```python
from build123d import *

# Parameters (mm, degrees)
BOSS_EXTRUDE1_DEPTH = 107.00004
SKETCH2_R           = 2
CUT_EXTRUDE1_DEPTH  = 16


with BuildPart() as part:
    # Sketch1 → Boss-Extrude1 (new body)
    with BuildSketch(Plane.XY):
        with BuildLine():
            Line((-6.5, 0), (6.5, 0))
            Line((6.5, 0), (6.5, 5.2))
            Line((6.5, 5.2), (4.8, 6.9))
            Line((4.8, 6.9), (4.8, 8.84))
            Line((4.8, 8.84), (5.754868434, 9.794868434))
            ThreePointArc((5.754868434, 9.794868434), (6.196913421, 10.683086579), (7.085131566, 11.125131566))
            Line((7.085131566, 11.125131566), (7.5, 11.54))
            Line((7.5, 11.54), (7.5, 12.85))
            Line((7.5, 12.85), (7.08164233, 13.26835767))
            ThreePointArc((7.08164233, 13.26835767), (6.196913421, 13.709913421), (5.75535767, 14.59464233))
            Line((5.75535767, 14.59464233), (5.35, 15))
            Line((5.35, 15), (-5.35, 15))
            Line((-5.35, 15), (-5.75535767, 14.59464233))
            ThreePointArc((-5.75535767, 14.59464233), (-6.196913421, 13.709913421), (-7.08164233, 13.26835767))
            Line((-7.08164233, 13.26835767), (-7.5, 12.85))
            Line((-7.5, 12.85), (-7.5, 11.54))
            Line((-7.5, 11.54), (-7.085131566, 11.125131566))
            ThreePointArc((-7.085131566, 11.125131566), (-6.196913421, 10.683086579), (-5.754868434, 9.794868434))
            Line((-5.754868434, 9.794868434), (-4.8, 8.84))
            Line((-4.8, 8.84), (-4.8, 6.9))
            Line((-4.8, 6.9), (-6.5, 5.2))
            Line((-6.5, 5.2), (-6.5, 0))
        make_face()
    extrude(amount=BOSS_EXTRUDE1_DEPTH)

    # Sketch2 → Cut-Extrude1 (cut, through all)
    with BuildSketch(Plane(origin=(0, 15, 0), x_dir=(1, 0, 0), z_dir=(0, 1, 0))):
        with Locations((0, -20)):
            Circle(SKETCH2_R)
        with Locations((0, -79.944)):
            Circle(SKETCH2_R)
    extrude(amount=-CUT_EXTRUDE1_DEPTH, mode=Mode.SUBTRACT)


solid = part.part
```
Design review of the part built by this model. Coordinates are the model's own, in mm. A direction names the side the tool comes from. Coordinates: 2 decimals unless noted, no trailing zeros. Order: outer loops, then holes, each group sorted by start corner. A loop starts at its lowest first (then second) coordinate and runs counter-clockwise, first axis right, second up. Notation, with made-up numbers: (-6, 47.25) -> (53, 47.25) arc R17 ccw to (53, 74.25) -> close; hole circle Ø5 at (-22, 45). An arc over 180 degrees is marked (long way). One line per item, written item: value. Start each with the question number.
Q1. Take a section at B-B, the plane z = 20. State the section outline as (x, y) points, then the cut area to 3 significant figures.
Q2. Take a section at D-D, the plane y = 1.25. State the section outline as (x, z) points.
Q3. Take a section at C-C, the plane z = 41. State the section outline as (x, y) points.
Q4. Take a section at A-A, the plane x = 0. State the section outline as (y, z) points.
Q5. Mouldability with a two-part tool opening along Y and no side actions: class faces 5 (the flat face through (0, 0, 53)), 6 (the flat face through (-4.8, 8, 53)), 7 (the flat face through (0, 15, 53)), 8 (the flat face through (-6.5, 3, 53)) as pulls with the +Y half, pulls with the -Y half, needs draft (parallel to the pull), parting line crosses it, or undercut.
Q6. Tool access review of faces 1 (the flat face through (0, 8, 0)), 2 (the flat face through (-5.6, 6.1, 52.8)), 3 (the flat face through (5.7, 6, 52.8)), 4 (the flat face through (6.5, 3, 53)): name each direction out of +Z, -Z, +X, -X, +Y, -Y from which nothing blocks a thin tool from reaching the whole face with its end or side.
Q7. For probe 1 along Z at (x, y) = (0, 4); probe 2 along Z at (x, y) = (0.5, 6.5); probe 3 along X at (y, z) = (8.5, 76), list the stretches that pass through material, from the lowest coordinate up.
Q8. Insertion check: pin 1 Ø5 at (y, z) = (5.5, 30.5) entering from +X; pin 2 Ø1.5 at (y, z) = (7, 51.5) entering from +X; pin 3 Ø0.6 at (y, z) = (7.5, 76) entering from -X. Each pin has a flat end and moves straight along its axis. Give the tip position at first contact, or say it passes through.
Values follow:
1. outline: (-7.5, 11.54) -> (-7.09, 11.13) arc R1.56 cw to (-5.75, 9.79) -> (-4.8, 8.84) -> (-4.8, 6.9) -> (-6.5, 5.2) -> (-6.5, 0) -> (-2, 0) -> (-2, 15) -> (-5.35, 15) -> (-5.76, 14.59) arc R1.56 cw to (-7.08, 13.27) -> (-7.5, 12.85) -> close; (2, 0) -> (6.5, 0) -> (6.5, 5.2) -> (4.8, 6.9) -> (4.8, 8.84) -> (5.75, 9.79) arc R1.56 cw to (7.09, 11.13) -> (7.5, 11.54) -> (7.5, 12.85) -> (7.08, 13.27) arc R1.56 cw to (5.76, 14.59) -> (5.35, 15) -> (2, 15) -> close
1. area: 124 mm2
2. outline: (-6.5, 0) -> (6.5, 0) -> (6.5, 107) -> (-6.5, 107) -> close; hole circle Ø4 at (0, 20); hole circle Ø4 at (0, 79.94)
3. outline: (-7.5, 11.54) -> (-7.09, 11.13) arc R1.56 cw to (-5.75, 9.79) -> (-4.8, 8.84) -> (-4.8, 6.9) -> (-6.5, 5.2) -> (-6.5, 0) -> (6.5, 0) -> (6.5, 5.2) -> (4.8, 6.9) -> (4.8, 8.84) -> (5.75, 9.79) arc R1.56 cw to (7.09, 11.13) -> (7.5, 11.54) -> (7.5, 12.85) -> (7.08, 13.27) arc R1.56 cw to (5.76, 14.59) -> (5.35, 15) -> (-5.35, 15) -> (-5.76, 14.59) arc R1.56 cw to (-7.08, 13.27) -> (-7.5, 12.85) -> close
4. outline: (0, 0) -> (15, 0) -> (15, 18) -> (0, 18) -> close; (0, 22) -> (15, 22) -> (15, 77.94) -> (0, 77.94) -> close; (0, 81.94) -> (15, 81.94) -> (15, 107) -> (0, 107) -> close
5. face 5: pulls with the -Y half
5. face 6: undercut
5. face 7: pulls with the +Y half
5. face 8: needs draft
6. face 1: -Z, +X, -X, +Y, -Y
6. face 2: +Z, -Z, -X
6. face 3: +Z, -Z, +X
6. face 4: +Z, -Z, +X, -Y
7. probe 1: z = 0 to 18, 22 to 77.94, 81.94 to 107
7. probe 2: z = 0 to 18.06, 21.94 to 78.01, 81.88 to 107
7. probe 3: x = -4.8 to 4.8
8. pin 1: stops at x = 6.5
8. pin 2: stops at x = 5.45
8. pin 3: stops at x = -4.8
